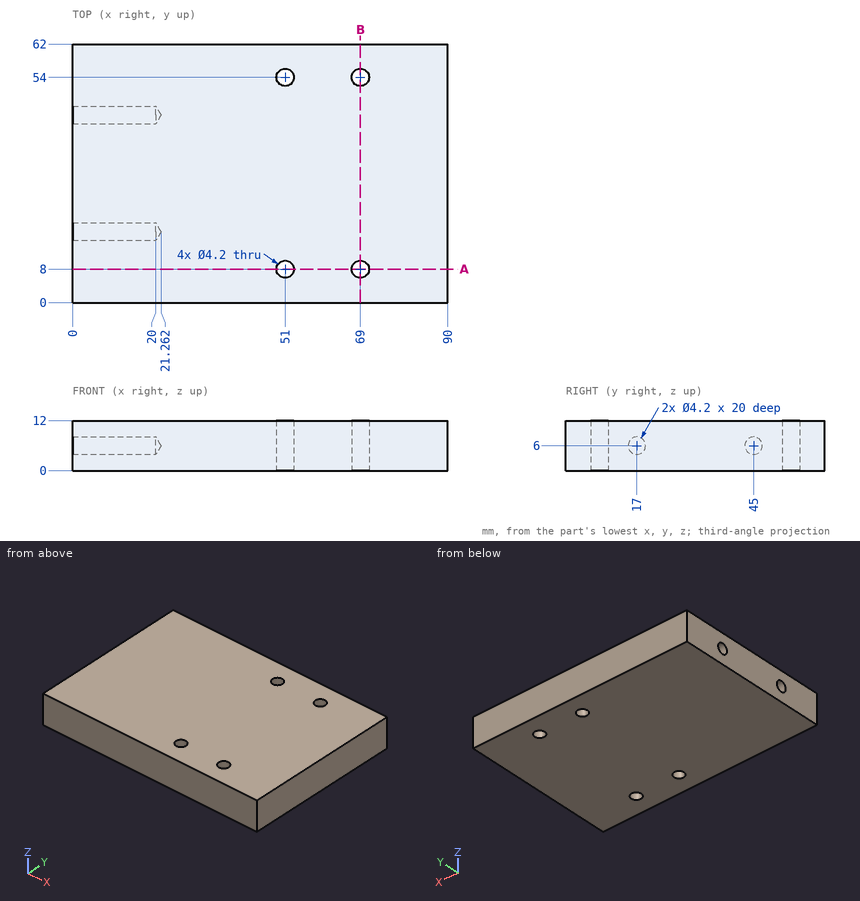
Source: three-view drawing plus pictorial views. Frame: mm from the lowest corner of the part. Give positions to 0.01 mm unless a question says otherwise; leave off trailing zeros. Write each loop counter-clockwise with the first axis right and the second up, starting at its lowest first coordinate (ties: lowest second). Pieces come first, ordered by that corner, then holes. Notation, with made-up numbers: (60, 50.25) -> (80, 50.25) arc R13 ccw to (80, 56.25) -> close; hole circle Ø8 at (82, -10.75). An arc over 180 degrees is marked (long way). Write item = value, one per line.
Q1. Cut plane B-B on x = 69. Return loops of the section in (y, z), then the cut area to 3 significant figures.
Here are the results:
outline = (0, 0) -> (5.9, 0) -> (5.9, 12) -> (0, 12) -> close; (10.1, 0) -> (51.9, 0) -> (51.9, 12) -> (10.1, 12) -> close; (56.1, 0) -> (62, 0) -> (62, 12) -> (56.1, 12) -> close
area = 643 mm²
Q2. Cut plane A-A on y = 8. Return loops of the section in (x, z).
Here are the results:
outline = (0, 0) -> (48.9, 0) -> (48.9, 12) -> (0, 12) -> close; (53.1, 0) -> (66.9, 0) -> (66.9, 12) -> (53.1, 12) -> close; (71.1, 0) -> (90, 0) -> (90, 12) -> (71.1, 12) -> close
Q3. Line query: line 1 (Y direction, x = 8.75, z = 6); line 2 (Y direction, x = 69, z = 4.5); line 3 (X direction, y = 55.5, z = 4.75). Output: solid intervals per line, ascending. Write a range as from..to.
Here are the results:
line_1 = 0..14.9, 19.1..42.9, 47.1..62
line_2 = 0..5.9, 10.1..51.9, 56.1..62
line_3 = 0..49.53, 52.47..67.53, 70.47..90
Q4. First-contact query: pin 1 (3.5 mm diameter, centred on y = 45, z = 6, fed in from -X). Flat tip, straight axial feed; report the tip coordinate or a pass-through.
Here are the results:
pin_1 = 20.21
